The listing builds one solid part. Answer for the finished solid, in the listing's coordinates (mm). Face numbers are marked on the shaded views. A direction names the side the tool comes from. Coordinates: 2 decimals unless noted, no trailing zeros. Order: outer loops, then holes, each group sorted by start corner. A loop starts at its lowest first (then second) coordinate and runs counter-clockwise, first axis right, second up. Notation, with made-up numbers: (41.5, 27.25) -> (93.5, 27.25) arc R31 cw to (93.5, 58.25) -> close; hole circle Ø5 at (60.25, 10). An arc over 180 degrees is marked (long way). One line per question, with ' | ' between items.
from build123d import *

# Parameters (mm, degrees)
SKETCH1_W           = 21
SKETCH1_H           = 21
BOSS_EXTRUDE1_DEPTH = 15
CUT_EXTRUDE1_DEPTH  = 5
SKETCH3_W           = 21
SKETCH3_H           = 3.4
CUT_EXTRUDE2_DEPTH  = 15
FILLET1_R           = 1


with BuildPart() as part:
    # Sketch1 → Boss-Extrude1 (new body)
    with BuildSketch(Plane(origin=(0, 0, 0), x_dir=(1, 0, 0), z_dir=(0, 1, 0))):
        Rectangle(SKETCH1_W, SKETCH1_H)
    extrude(amount=BOSS_EXTRUDE1_DEPTH)

    # Sketch2 → Cut-Extrude1 (cut)
    with BuildSketch(Plane(origin=(0, 15, 0), x_dir=(1, 0, 0), z_dir=(0, 1, 0))):
        Polygon((-10.5, 6.325), (-5.5, 6.325), (-5.5, 8.575), (-2.85, 8.575), (-2.85, 0.925), (-5.5, 0.925), (-5.5, 3.175), (-10.5, 3.175), align=None)
        Polygon((10.5, 3.175), (10.5, 6.325), (5.5, 6.325), (5.5, 8.575), (2.85, 8.575), (2.85, 0.925), (5.5, 0.925), (5.5, 3.175), align=None)
        Polygon((-3.825, -2.85), (3.825, -2.85), (3.825, -5.5), (1.575, -5.5), (1.575, -10.5), (-1.575, -10.5), (-1.575, -5.5), (-3.825, -5.5), align=None)
    extrude(amount=-CUT_EXTRUDE1_DEPTH, mode=Mode.SUBTRACT)

    # Sketch3 → Cut-Extrude2 (cut)
    with BuildSketch(Plane.XY.offset(10.5)):
        with Locations((0, 3.7)):
            Rectangle(SKETCH3_W, SKETCH3_H)
    extrude(amount=-CUT_EXTRUDE2_DEPTH, mode=Mode.SUBTRACT)

    # Fillet1
    fillet1_edges = [part.edges().sort_by_distance(p)[0] for p in [
        (1.575, 12.5, 5.5),
        (-1.575, 12.5, 5.5),
        (-3.825, 15, 4.175),
        (-2.7, 15, 5.5),
        (-1.575, 15, 8),
        (1.575, 15, 8),
        (2.7, 15, 5.5),
        (3.825, 15, 4.175),
        (0, 15, 2.85),
        (10.5, 12.5, -3.175),
        (5.5, 12.5, -3.175),
        (5.5, 12.5, -6.325),
        (10.5, 12.5, -6.325),
        (8, 15, -3.175),
        (8, 15, -6.325),
        (5.5, 15, -7.45),
        (4.175, 15, -8.575),
        (2.85, 15, -4.75),
        (4.175, 15, -0.925),
        (5.5, 15, -2.05),
        (-10.5, 12.5, -3.175),
        (-10.5, 12.5, -6.325),
        (-5.5, 12.5, -6.325),
        (-5.5, 12.5, -3.175),
        (-8, 15, -3.175),
        (-5.5, 15, -2.05),
        (-4.175, 15, -0.925),
        (-2.85, 15, -4.75),
        (-4.175, 15, -8.575),
        (-5.5, 15, -7.45),
        (-8, 15, -6.325),
    ]]
    fillet(fillet1_edges, radius=FILLET1_R)


solid = part.part
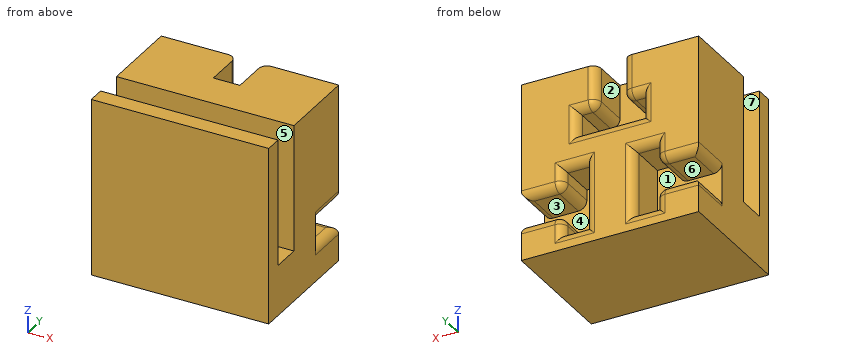
Item 1: Section A-A, the plane z = 7.25 is taken. Give the vertices of the cut face in (x, y) (3 decimals).
Computed values:
outline: (-10.5, 0) -> (10.5, 0) -> (10.5, 2) -> (-10.5, 2) -> close; (-10.5, 5.4) -> (10.5, 5.4) -> (10.5, 15) -> (2.575, 15) arc R1 ccw to (1.575, 14) -> (1.575, 10) -> (-1.575, 10) -> (-1.575, 14) arc R1 ccw to (-2.575, 15) -> (-10.5, 15) -> close
Item 2: Section D-D, the plane y = 3 is taken. Give the vertices of the cut face in (x, z), plus the area to 3 significant figures.
Computed values:
outline: (-10.5, -10.5) -> (10.5, -10.5) -> (10.5, -4.5) -> (-10.5, -4.5) -> close | area: 126 mm^2
Item 3: Section C-C, the plane z = 4.5 is taken. Give the vertices of the cut face in (x, y) (3 decimals), plus the area to 3 significant figures.
Computed values:
outline: (-10.5, 0) -> (10.5, 0) -> (10.5, 2) -> (-10.5, 2) -> close; (-10.5, 5.4) -> (10.5, 5.4) -> (10.5, 15) -> (4.825, 15) arc R1 ccw to (3.825, 14) -> (3.825, 10) -> (-3.825, 10) -> (-3.825, 14) arc R1 ccw to (-4.825, 15) -> (-10.5, 15) -> close | area: 205 mm^2
Item 4: Section B-B, the plane x = -7.25 is taken. Give the vertices of the cut face in (y, z) (3 decimals).
Computed values:
outline: (0, -10.5) -> (15, -10.5) -> (15, -7.325) arc R1 ccw to (14, -6.325) -> (10, -6.325) -> (10, -3.175) -> (14, -3.175) arc R1 ccw to (15, -2.175) -> (15, 10.5) -> (5.4, 10.5) -> (5.4, -4.5) -> (2, -4.5) -> (2, 10.5) -> (0, 10.5) -> close
Item 5: Each of these flat-tipped pins is pushed along its axis until it touches: pin 1 Ø2.5 at (x, z) = (0, 5) entering from +Y; pin 2 Ø1.2 at (y, z) = (12, -5) entering from +X; pin 3 Ø1.2 at (y, z) = (13, -4.5) entering from -X. Where does it stop, or does it pass through?
Computed values:
pin 1: stops at y = 10 | pin 2: stops at x = 2.85 | pin 3: stops at x = -2.85
Item 6: Determine the mould class of the marked faces 4, 5, 6 and 7 for opening direction Y: pulls with the +Y half, pulls with the -Y half, needs draft (parallel to the pull), parting line crosses it, or undercut.
Computed values:
face 4: pulls with the +Y half | face 5: undercut | face 6: needs draft | face 7: undercut
Item 7: For the marked faces 1, 2 and 3, determine the directions among +Z, -Z, +X, -X, +Y, -Y from which every point of the face is accessible in a straight line to the end or side of a thin tool.
Computed values:
face 1: +Y | face 2: +Z, +Y | face 3: +X, +Y
Item 8: Find the intervals of material crossed by L1, parallel to X at y = 13.25, z = -7.75; L2, parallel to Y at x = -7.75, z = -0.75; L3, parallel to Y at x = 0, z = 4.5, in increasing order.
Computed values:
L1: x = -10.5 to -5.5, -2.85 to 2.85, 5.5 to 10.5 | L2: y = 0 to 2, 5.4 to 15 | L3: y = 0 to 2, 5.4 to 10
